from build123d import *

# Parameters (mm, degrees)
CROQUIS1_W              = 13
CROQUIS1_H              = 13
SALIENTE_EXTRUIR1_DEPTH = 40
CORTAR_EXTRUIR1_REACH   = 43.043
CROQUIS2_W              = 12
CROQUIS2_H              = 12
CROQUIS4_R              = 12
CORTAR_EXTRUIR3_DEPTH   = 26


with BuildPart() as part:
    # Croquis1 → Saliente-Extruir1 (new body)
    with BuildSketch(Plane.XY):
        Rectangle(CROQUIS1_W, CROQUIS1_H)
    extrude(amount=SALIENTE_EXTRUIR1_DEPTH)

    # Croquis2 → Cortar-Extruir1 (cut, up to next)
    with BuildSketch(Plane.XY.offset(40), mode=Mode.PRIVATE) as cortar_extruir1_sk1:
        Rectangle(CROQUIS2_W, CROQUIS2_H)
    cortar_extruir1_tool1 = extrude(cortar_extruir1_sk1.sketch, amount=-CORTAR_EXTRUIR1_REACH, mode=Mode.PRIVATE) & part.part
    add(cortar_extruir1_tool1.solids().sort_by_distance((0, 0, 40))[0], mode=Mode.SUBTRACT)

    # Croquis4 → Cortar-Extruir3 (cut)
    with BuildSketch(Plane(origin=(0, 6.5, 0), x_dir=(1, 0, 0), z_dir=(0, 1, 0))):
        with Locations((0, -40)):
            Circle(CROQUIS4_R)
    extrude(amount=-CORTAR_EXTRUIR3_DEPTH, mode=Mode.SUBTRACT)


solid = part.part
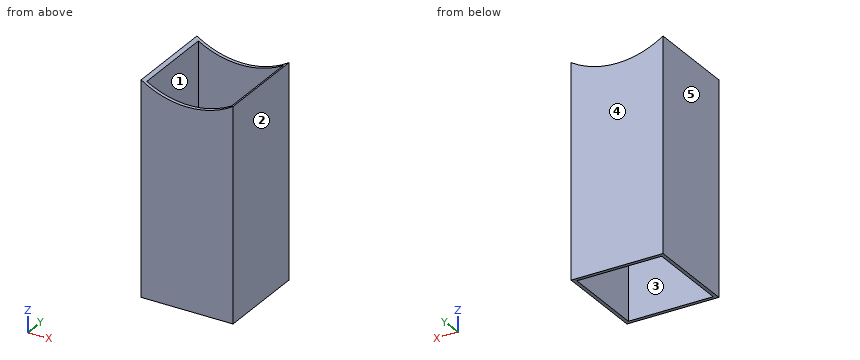
Input: part model. Units: mm. Frame: model coordinates. Face numbers are marked on the shaded views. A direction names the side the tool comes from. Coordinates: 2 decimals unless noted, no trailing zeros. Loops run counter-clockwise (first coordinate to the right, second up) from the corner with the lowest first, then second, coordinate; pieces in that order, holes last.
(1) Material intervals for probe 1 along Y at (x, z) = (5.25, 9.5), sorted ascending.
(2) Section C-C on x = 0.25. Return the cut outline in (y, z), then the cut area to 3 significant figures.
(3) Set-up query: the marked faces 1 and 2. Return all of +Z, -Z, +X, -X, +Y, -Y with unobstructed straight access to the full face (end or side cutting, diameter ignored); none if empty.
(4) Section B-B on y = 1. Return the cut outline in (x, z), then the cut area to 3 significant figures.
(5) Pull-direction query (X, two-part tool) for the marked faces 3, 4 and 5; classes: released by +X, released by -X, zero draft, split by the parting line, or undercut.
(6) Section A-A on z = 15.5. Return the cut outline in (x, y), then the cut area to 3 significant figures.
Data:
1. probe 1: y = -6.5 to -6, 6 to 6.5
2. outline: (-6.5, 0) - (-6, 0) - (-6, 28) - (-6.5, 28) - close; (6, 0) - (6.5, 0) - (6.5, 28) - (6, 28) - close
2. area: 28.0 mm2
3. face 1: +Z, -Z
3. face 2: +Z, -Z, +X, +Y, -Y
4. outline: (-6.5, 0) - (-6, 0) - (-6, 29.61) arc R12 cw to (-6.5, 29.91) - close; (6, 0) - (6.5, 0) - (6.5, 29.91) arc R12 cw to (6, 29.61) - close
4. area: 29.8 mm2
5. face 3: undercut
5. face 4: zero draft
5. face 5: released by -X
6. outline: (-6.5, -6.5) - (6.5, -6.5) - (6.5, 6.5) - (-6.5, 6.5) - close; hole (-6, -6) - (6, -6) - (6, 6) - (-6, 6) - close
6. area: 25.0 mm2
